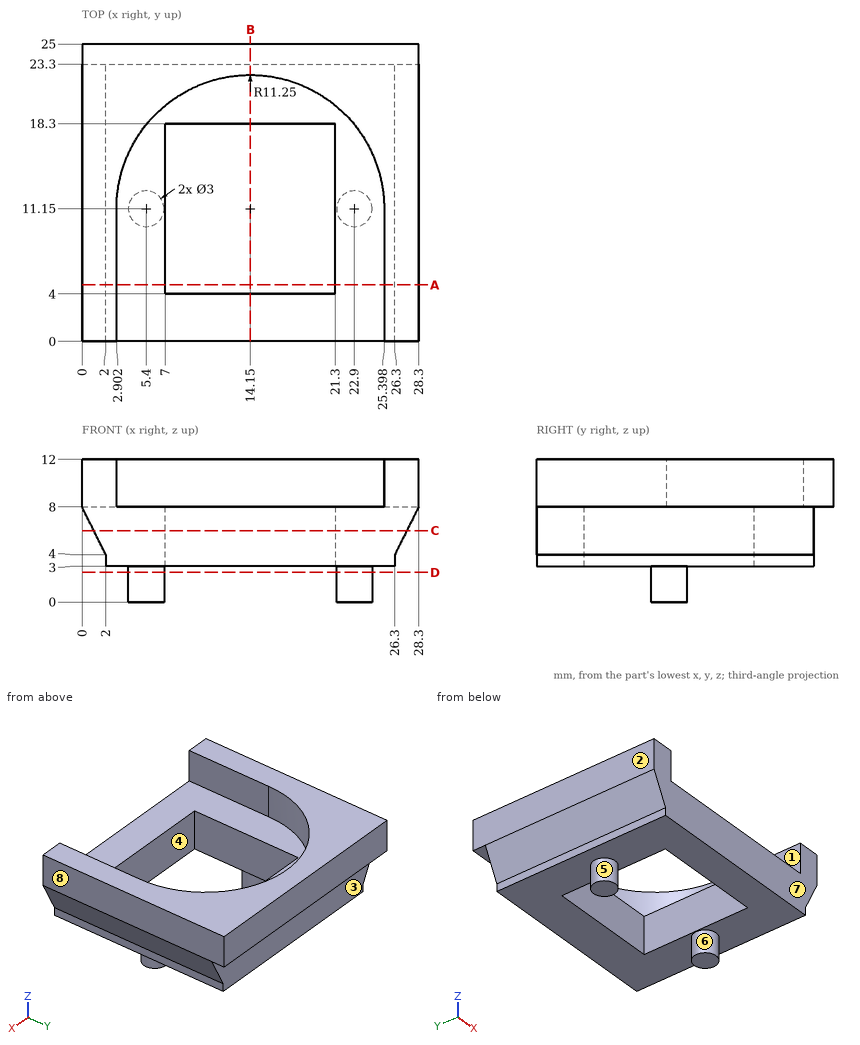
Geometry check sheet. Reference: drawing and pictorial views, mm from the part's lowest x, y, z. A direction names the side the tool comes from. Round coordinates to 2 decimals unless told otherwise and drop trailing zeros. Order: outer loops, then holes, each group sorted by start corner. A loop starts at its lowest first (then second) coordinate and runs counter-clockwise, first axis right, second up. Notation, with made-up numbers: (40.5, 36) - (57.5, 36) arc R18 ccw to (57.5, 42) - close; hole circle Ø3 at (3.25, 49). An arc over 180 degrees is marked (long way). Use a Markdown table: item, result. Add a question column.
1) Section check A-A (y = 4.75). Record the cut outline in (x, z), then the cut area to 3 significant figures.
2) Section check D-D (z = 2.5). Record the cut outline in (x, y), then the cut area to 3 significant figures.
3) Mould release check, pull along X, two halves, no side actions. Record for the marked faces 6, 7 and 8: released by +X, released by -X, zero draft, split by the parting line, or undercut.
4) Section check C-C (z = 6). Record the cut outline in (x, y).
5) Gauge pin test, flat ends, axial feed: P1, Ø1.1, axis at y = 12, z = 3.5, coming from the +X side (3 decimals); P2, Ø5, axis at y = 13, z = 5, coming from the -X side; P3, Ø5, axis at x = 8.5, y = 5.5, coming from the +Z side; P4, Ø3, axis at x = 14, y = 16.5, coming from the -Z side. Record the tip position at first contact, or that the pin passes through.
6) Thickness scan on line 1 along X through (y, z) = (4.75, 11.75); line 2 along Y through (x, z) = (18.75, 7); line 3 along Z through (x, y) = (23.75, 4.5). Record the ranges inside material, lowest first.
7) Set-up check for the marked faces 1, 2, 3, 4 and 5: record each of +Z, -Z, +X, -X, +Y, -Y from which the full face is reachable in a straight line by a thin tool's end or side.
8) Section check B-B (x = 14.15). Record the cut outline in (y, z).
Established:
| question | item | result |
|---|---|---|
| 1 | outline | (0, 8) - (2, 4) - (2, 3) - (7, 3) - (7, 8) - (2.9, 8) - (2.9, 12) - (0, 12) - close; (21.3, 3) - (26.3, 3) - (26.3, 4) - (28.3, 8) - (28.3, 12) - (25.4, 12) - (25.4, 8) - (21.3, 8) - close |
| 1 | area | 81.2 mm2 |
| 2 | outline | circle Ø3 at (5.4, 11.15); circle Ø3 at (22.9, 11.15) |
| 2 | area | 14.1 mm2 |
| 3 | face 6 | undercut |
| 3 | face 7 | zero draft |
| 3 | face 8 | released by +X |
| 4 | outline | (1, 0) - (27.3, 0) - (27.3, 23.3) - (1, 23.3) - close; hole (7, 4) - (21.3, 4) - (21.3, 18.3) - (7, 18.3) - close |
| 5 | P1 | x = 26.325 |
| 5 | P2 | x = 0.25 |
| 5 | P3 | z = 8 |
| 5 | P4 | through |
| 6 | line 1 | 0 to 2.9, 25.4 to 28.3 |
| 6 | line 2 | 0 to 4, 18.3 to 23.3 |
| 6 | line 3 | 3 to 8 |
| 7 | face 1 | +Z, -Y |
| 7 | face 2 | +Z, -Z, -X, +Y, -Y |
| 7 | face 3 | -Z, +X, -X, +Y |
| 7 | face 4 | +Z, -Z |
| 7 | face 5 | -Z |
| 8 | outline | (0, 3) - (4, 3) - (4, 8) - (0, 8) - close; (18.3, 3) - (23.3, 3) - (23.3, 8) - (25, 8) - (25, 12) - (22.4, 12) - (22.4, 8) - (18.3, 8) - close |
